Job drawing, mm, ordinate dimensions from the low corner. One solid piece. Give positions to 0.01 mm unless a question says otherwise; leave off trailing zeros. Order: outer loops, then holes, each group sorted by start corner. A loop starts at its lowest first (then second) coordinate and runs counter-clockwise, first axis right, second up. Notation, with made-up numbers: (35, 54) -> (57, 54) arc R25 cw to (57, 67) -> close; hole circle Ø5 at (58, 76.5). An arc over 180 degrees is marked (long way). Write item = value, one per line. Start each with the question number.
(1) Saw through at D-D, the plane x = 58.5. List the corners of the cut face in (y, z).
(2) Two-plate mould, pull along Y, no slides. Class the marked faces 1, 2 and 3: pulls with the +Y half, pulls with the -Y half, needs draft (parallel to the pull), parting line crosses it, or undercut.
(3) Probe line 1 along Y through (x, z) = (74.4, 4); line 2 along Y through (x, z) = (28.5, 6); line 3 along X through (y, z) = (15.5, 0.5). List the from-to ranges inside material, lowest first. Write a range as from..to.
(4) Saw through at C-C, the plane z = 4.75. List the corners of the cut face in (x, y).
(5) Saw through at B-B, the plane x = 6.9. List the corners of the cut face in (y, z).
(6) Saw through at A-A, the plane y = 11.5. List the corners of the cut face in (x, z), then the cut area to 3 significant figures.
(7) Flat gauge pins, fed straight in: pin 1 (3 mm diameter, centred on x = 6.9, y = 11.5, fed in from -Z); pin 2 (4 mm diameter, centred on x = 37, y = 17, fed in from -Z); pin 3 (3 mm diameter, centred on x = 53, z = 2.5, fed in from +Y); pin 4 (2 mm diameter, centred on y = 20, z = 1, fed in from +X). Where does each tip first touch, or does it go through?
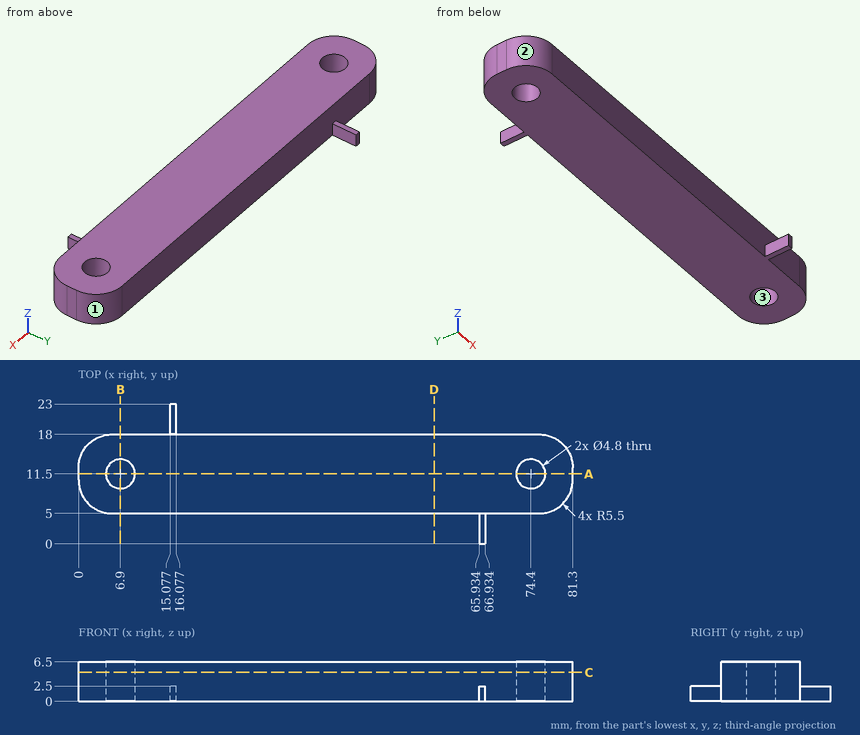
Results list:
q1.outline = (5, 0) -> (18, 0) -> (18, 6.5) -> (5, 6.5) -> close
q2.face_1 = pulls with the +Y half
q2.face_2 = pulls with the -Y half
q2.face_3 = undercut
q3.line_1 = 5..9.1, 13.9..18
q3.line_2 = 5..18
q3.line_3 = 0.89..80.41
q4.outline = (0, 10.5) arc R5.5 ccw to (5.5, 5) -> (75.8, 5) arc R5.5 ccw to (81.3, 10.5) -> (81.3, 12.5) arc R5.5 ccw to (75.8, 18) -> (5.5, 18) arc R5.5 ccw to (0, 12.5) -> close; hole circle Ø4.8 at (6.9, 11.5); hole circle Ø4.8 at (74.4, 11.5)
q5.outline = (5, 0) -> (9.1, 0) -> (9.1, 6.5) -> (5, 6.5) -> close; (13.9, 0) -> (18, 0) -> (18, 6.5) -> (13.9, 6.5) -> close
q6.outline = (0, 0) -> (4.5, 0) -> (4.5, 6.5) -> (0, 6.5) -> close; (9.3, 0) -> (72, 0) -> (72, 6.5) -> (9.3, 6.5) -> close; (76.8, 0) -> (81.3, 0) -> (81.3, 6.5) -> (76.8, 6.5) -> close
q6.area = 466 mm^2
q7.pin_1 = through
q7.pin_2 = 0
q7.pin_3 = 18
q7.pin_4 = 16.08
